```python
from build123d import *

# Parameters (mm, degrees)
SKETCH_R        = 73
SKETCH_R_2      = 2.5
PAD_DEPTH       = 3
SKETCH002_R     = 1.75
POCKET_DEPTH    = 3.001
SKETCH003_R     = 1.25
POCKET001_DEPTH = 3.001


with BuildPart() as part:
    # Sketch → Pad (new body)
    with BuildSketch(Plane.XY):
        Circle(SKETCH_R)
        with Locations((0, 67)):
            Circle(SKETCH_R_2, mode=Mode.SUBTRACT)
    extrude(amount=PAD_DEPTH)

    # Sketch002 (on Face4 of Pad) → Pocket (cut, through all)
    with BuildSketch(Plane.XY.offset(3)):
        with Locations((-40, -52.497619)):
            Circle(SKETCH002_R)
        with Locations((40, -52.497619)):
            Circle(SKETCH002_R)
        with Locations((-50, 43.081318)):
            Circle(SKETCH002_R)
        with Locations((50, 43.081318)):
            Circle(SKETCH002_R)
    extrude(amount=-POCKET_DEPTH, mode=Mode.SUBTRACT)

    # Sketch003 (on Face3 of Pocket) → Pocket001 (cut, through all)
    with BuildSketch(Plane.XY.offset(3)):
        with Locations((-23, 45)):
            Circle(SKETCH003_R)
        with Locations((-23, -30)):
            Circle(SKETCH003_R)
        with Locations((0, 45)):
            Circle(SKETCH003_R)
        with Locations((0, -30)):
            Circle(SKETCH003_R)
        with Locations((23, 45)):
            Circle(SKETCH003_R)
        with Locations((23, -30)):
            Circle(SKETCH003_R)
        with BuildLine():
            ThreePointArc((-7, -56.5), (-10.5, -60), (-7, -63.5))
            Line((-7, -63.5), (7, -63.5))
            ThreePointArc((7, -63.5), (10.5, -60), (7, -56.5))
            Line((-7, -56.5), (7, -56.5))
        make_face()
    extrude(amount=-POCKET001_DEPTH, mode=Mode.SUBTRACT)


solid = part.part
```
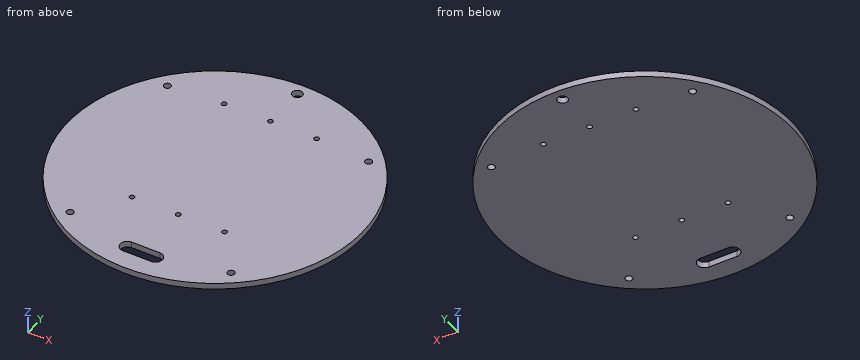
Read the model definition and answer for the solid it produces. Units are mm, in the model's axes. Coordinates: 2 decimals unless noted, no trailing zeros. Loops run counter-clockwise (first coordinate to the right, second up) from the corner with the lowest first, then second, coordinate; pieces in that order, holes last. Notation, with made-up numbers: (57, -10.5) -> (99, -10.5) arc R26 ccw to (99, 7.5) -> close; hole circle Ø10 at (-24, 68.5). An arc over 180 degrees is marked (long way). Return JSON: item names as keys, results as strings.
Item 1: Find section D-D (y = 13). Determine the outline of the cut face in (x, z), plus the area to 3 significant figures.
Answers:
{"outline": "(-71.83, 0) -> (71.83, 0) -> (71.83, 3) -> (-71.83, 3) -> close", "area": "431 mm2"}
Item 2: Flat-ended cylindrical pins translate along their axes: P1, Ø3, axis at x = 23, y = -30, coming from the +Z side; P2, Ø1, axis at x = -34.5, z = 2.5, coming from the +Y side. Find the tip coordinate at first contact, or state that the pin passes through.
Answers:
{"P1": "stops at z = 3", "P2": "stops at y = 64.6"}
Item 3: Find section A-A (x = 40). Determine the outline of the cut face in (y, z).
Answers:
{"outline": "(-61.07, 0) -> (-54.25, 0) -> (-54.25, 3) -> (-61.07, 3) -> close; (-50.75, 0) -> (61.07, 0) -> (61.07, 3) -> (-50.75, 3) -> close"}
Item 4: Find section C-C (y = -20.5). Determine the outline of the cut face in (x, z), plus the area to 3 significant figures.
Answers:
{"outline": "(-70.06, 0) -> (70.06, 0) -> (70.06, 3) -> (-70.06, 3) -> close", "area": "420 mm2"}
Item 5: Find section B-B (z = 2.3). Count the separate pieces of the cut face and the enclosed holes in it, plus the area to 3 significant figures.
Answers:
{"separate pieces": "1", "enclosed holes": "12", "area": "16,500 mm2"}
Item 6: Find the intervals of material crossed by probe 1 along X at (y, z) = (-51, 2.2); probe 2 along X at (y, z) = (-31, 0.5); probe 3 along Y at (x, z) = (50, 1.5), in increasing order.
Answers:
{"probe 1": "x = -52.23 to -40.91, -39.09 to 39.09, 40.91 to 52.23", "probe 2": "x = -66.09 to -23.75, -22.25 to -0.75, 0.75 to 22.25, 23.75 to 66.09", "probe 3": "y = -53.19 to 41.33, 44.83 to 53.19"}
